from build123d import *

# Parameters (mm, degrees)
SKIZZE1_R                                            = 20.5
SKIZZE1_R_2                                          = 7
AUFSATZ_LINEAR_AUSTRAGEN1_DEPTH                      = 5
SKIZZE3_R                                            = 30
SKIZZE3_R_2                                          = 7
AUFSATZ_LINEAR_AUSTRAGEN2_DEPTH                      = 4
DURCHGANGSLOCH_F_R_M41_D                             = 4.5
STIRNSENKUNG_F_R_M4_ZYLINDERSCHRAUBE_MIT_D           = 4.5
STIRNSENKUNG_F_R_M4_ZYLINDERSCHRAUBE_MIT_CBORE_D     = 8
STIRNSENKUNG_F_R_M4_ZYLINDERSCHRAUBE_MIT_CBORE_DEPTH = 4.4
FASE1_SIZE                                           = 0.25


with BuildPart() as part:
    # Skizze1 → Aufsatz-Linear austragen1 (new body)
    with BuildSketch(Plane(origin=(0, 0, 0), x_dir=(1, 0, 0), z_dir=(0, 1, 0))):
        with Locations(Location((0, 0, 0), (0, 0, 270))):
            Circle(SKIZZE1_R)
        with Locations(Location((0, 0, 0), (0, 0, 270))):
            Circle(SKIZZE1_R_2, mode=Mode.SUBTRACT)
    extrude(amount=AUFSATZ_LINEAR_AUSTRAGEN1_DEPTH)

    # Skizze3 → Aufsatz-Linear austragen2 (add)
    with BuildSketch(Plane(origin=(0, 5, 0), x_dir=(1, 0, 0), z_dir=(0, 1, 0))):
        with Locations(Location((0, 0, 0), (0, 0, 270))):
            Circle(SKIZZE3_R)
        with Locations(Location((0, 0, 0), (0, 0, 270))):
            Circle(SKIZZE3_R_2, mode=Mode.SUBTRACT)
    extrude(amount=AUFSATZ_LINEAR_AUSTRAGEN2_DEPTH)

    # Durchgangsloch für M41 (through all)
    with Locations(Plane(origin=(0, 5, 0), x_dir=(-1, 0, 0), z_dir=(0, -1, 0))):
        with Locations((0, 25), (-25, 0), (0, -25), (25, 0)):
            Hole(DURCHGANGSLOCH_F_R_M41_D / 2)

    # Stirnsenkung für M4 Zylinderschraube mit Innensechskant1 (through all)
    with Locations(Plane(origin=(0, 9, 0), x_dir=(1, 0, 0), z_dir=(0, 1, 0))):
        with Locations((-10.392304845, 6), (0, 12), (10.392304845, 6), (10.392304845, -6), (0, -12), (-10.392304845, -6)):
            CounterBoreHole(STIRNSENKUNG_F_R_M4_ZYLINDERSCHRAUBE_MIT_D / 2, STIRNSENKUNG_F_R_M4_ZYLINDERSCHRAUBE_MIT_CBORE_D / 2, STIRNSENKUNG_F_R_M4_ZYLINDERSCHRAUBE_MIT_CBORE_DEPTH)

    # Fase1
    fase1_edges = [part.edges().sort_by_distance(p)[0] for p in [
        (0, 9, -30),
        (0, 5, -30),
        (0, 9, -7),
        (-27.25, 5, 0),
        (-27.25, 9, 0),
        (-2.25, 5, 25),
        (-2.25, 9, 25),
        (22.75, 5, 0),
        (22.75, 9, 0),
        (-2.25, 5, -25),
        (-2.25, 9, -25),
        (-14.392304845, 9, -6),
        (0, 5, -20.5),
        (-14.392304845, 9, 6),
        (-4, 9, 12),
        (6.392304845, 9, 6),
        (6.392304845, 9, -6),
        (-4, 9, -12),
    ]]
    chamfer(fase1_edges, length=FASE1_SIZE)


solid = part.part
Can you work these out from the model? Positions are in its coordinate system, mm. A direction names the side the tool comes from. Coordinates: 2 decimals unless noted, no trailing zeros. Loops run counter-clockwise (first coordinate to the right, second up) from the corner with the lowest first, then second, coordinate; pieces in that order, holes last. Notation, with made-up numbers: (43, 14) - (91, 14) arc R23 cw to (91, 43) - close; hole circle Ø2 at (29.25, -21.5). An arc over 180 degrees is marked (long way). Put each result on its own line as item: value. Start each with the question number.
Item 1: If we mould it in two halves opening along X, with no side actions, what happens to faces 1 (the face through (-9, 0, 0)), 2 (the face through (12.64, 2.27, 5.9))? For each: +X half, -X half, draft (parallel to the pull), parting line (faces both ways), or undercut.
Item 2: Suppose I cut it at B-B (y = 1.75). Please give me the cut outline in (x, z).
Item 3: For pin 1 (3 mm diameter, centred on x = 19, y = 2.5, fed in from -Z); pin 2 (4 mm diameter, centred on x = 15, y = 2.5, fed in from +Z); pin 3 (7 mm diameter, centred on x = 25, z = 0, fed in from -Y), each with a flat end and sliding along its axis, tell me the tip position at first contact or that it passes through.
Item 4: Which directions (+Z, -Z, +X, -X, +Y, -Y) give clear straight access to the entire face, cutting with the end or side of a thin tool? Please do faces 3 (the face through (9.5, 6.7, -2.1)), 4 (the face through (-22.854, 7.025, -0.676)).
Item 5: Suppose I cut it at A-A (y = 8). State how many separate pieces and enclosed holes the cut face has, and give its area (3 significant figures).
Item 6: If I drill on line 1 along X through (y, z) = (6.65, 12); line 2 along X through (y, z) = (7.4, 6); line 3 along Z through (x, y) = (-1, 2.5), over which ranges is the centre line in solid material (lowest first)?
Here are the results:
1. face 1: draft
1. face 2: undercut
2. outline: circle Ø41 at (0, 0); hole circle Ø4.5 at (-10.39, -6); hole circle Ø4.5 at (-10.39, 6); hole circle Ø14 at (0, 0); hole circle Ø4.5 at (0, -12); hole circle Ø4.5 at (0, 12); hole circle Ø4.5 at (10.39, -6); hole circle Ø4.5 at (10.39, 6)
3. pin 1: z = -10.68
3. pin 2: z = 15.85
3. pin 3: y = 5
4. face 3: +Y
4. face 4: +Y, -Y
5. separate pieces: 1
5. enclosed holes: 11
5. area: 2,310 mm²
6. line 1: -27.5 to -4, 4 to 27.5
6. line 2: -29.39 to -14.39, -6.39 to -3.61, 3.61 to 6.39, 14.39 to 29.39
6. line 3: -20.48 to -14.02, -9.98 to -6.93, 6.93 to 9.98, 14.02 to 20.48
